from build123d import *

# Parameters (mm, degrees)
F0_W     = 25
F0_H     = 43
F1_DEPTH = 5
F2_R     = 1
F3_DEPTH = 5.001
F4_R     = 5
F5_R     = 2.49999
F6_R     = 3
F7_DEPTH = 2


# Not quite as in the source:
# - a fillet or chamfer is up to 0.001 mm smaller than in the source, because OpenCascade refuses the exact size


with BuildPart() as f1:
    # F0 (on Top) → F1 (new body)
    with BuildSketch(Plane.XY):
        with Locations((0, 21.5)):
            Rectangle(F0_W, F0_H)
    extrude(amount=-F1_DEPTH)

    # F2 (on face) → F3 (cut, through all)
    with BuildSketch(Plane.XY):
        with Locations((0, 37)):
            Circle(F2_R)
        with Locations((0, 23)):
            Circle(F2_R)
    extrude(amount=-F3_DEPTH, mode=Mode.SUBTRACT)

    # F4
    f4_edges = [f1.edges().sort_by_distance(p)[0] for p in [
        (-12.5, 43, -2.5),
        (12.5, 43, -2.5),
    ]]
    fillet(f4_edges, radius=F4_R)

    # F5 (radius 2.5 in the source; OpenCascade refuses exactly that, so slightly less here)
    f5_edges = [f1.edges().sort_by_distance(p)[0] for p in [
        (-12.5, 19, 0),
        (-12.5, 19, -5),
    ]]
    fillet(f5_edges, radius=F5_R)

    # F6 (on face) → F7 (cut)
    with BuildSketch(Plane(origin=(0, 0, -5), x_dir=(1, 0, 0), z_dir=(0, 0, -1))):
        with Locations((0, -37)):
            Circle(F6_R)
        with Locations((0, -23)):
            Circle(F6_R)
    extrude(amount=-F7_DEPTH, mode=Mode.SUBTRACT)

    # F8: F1 across plane


with BuildPart() as f1_1:
    add(f1.part)
    add(f1.part.mirror(Plane.XZ))


solid = f1_1.part
Check sheet for the modelled part. Datum: model origin and axes. Units: mm. A direction names the side the tool comes from. Coordinates: 2 decimals unless noted, no trailing zeros. Write each loop counter-clockwise with the first axis right and the second up, starting at its lowest first coordinate (ties: lowest second). Pieces come first, ordered by that corner, then holes.
Item 1: Cross-section at B-B on z = -1.65. Record the boundary of the cut face in (x, y).
Numbers:
outline: (-12.35, -38) arc R4.85 ccw to (-7.5, -42.85) - (7.5, -42.85) arc R4.85 ccw to (12.35, -38) - (12.35, 38) arc R4.85 ccw to (7.5, 42.85) - (-7.5, 42.85) arc R4.85 ccw to (-12.35, 38) - close; hole circle Ø2 at (0, -37); hole circle Ø2 at (0, -23); hole circle Ø2 at (0, 23); hole circle Ø2 at (0, 37)
Item 2: Scan lines: probe 1 along Y at (x, z) = (0, -3.7); probe 2 along Y at (x, z) = (0, -4.45); probe 3 along Z at (x, y) = (10.25, 8.5). Record each from-to range of solid material in increasing order.
Numbers:
probe 1: y = -42.69 to -40, -34 to -26, -20 to 20, 26 to 34, 40 to 42.69
probe 2: y = -42.06 to -40, -34 to -26, -20 to 20, 26 to 34, 40 to 42.06
probe 3: z = -4.99 to -0.01
Item 3: Depth check by flat-ended pin: pin 1 Ø1.8 at (x, y) = (-1, 23.5) entering from -Z. Enter the tip coordinate at first touch or a pass-through.
Numbers:
pin 1: stops at z = -3
Item 4: Cross-section at C-C on x = 0. Count the separate pieces of the cut face and the enclosed holes in it, then the cut area to 3 significant figures.
Numbers:
separate pieces: 5
enclosed holes: 0
area: 353 mm2
Item 5: Access from +Z, -Z, +X, -X, +Y, -Y to the whole of each face (thin tool, end or side, straight path). Record for faces 5 (the face through (-12, -1, -1)), 6 (the face through (-1, -36, -3)).
Numbers:
face 5: +Z, -X, +Y, -Y
face 6: -Z
Item 6: Mould release check, pull along X, two halves, no side actions. Record for faces 1 (the face through (12, 1, -4)), 2 (the face through (-0.65, -25.93, -4.01)), 3 (the face through (-1, 22, -3)), 4 (the face through (0.105, -42.287, -0.752)): released by +X, released by -X, zero draft, split by the parting line, or undercut.
Numbers:
face 1: released by +X
face 2: undercut
face 3: undercut
face 4: zero draft
